Geometry: final body of the model. Coordinates: model frame, mm. A direction names the side the tool comes from. Give positions to 0.01 mm unless a question says otherwise; leave off trailing zeros. Loops run counter-clockwise (first coordinate to the right, second up) from the corner with the lowest first, then second, coordinate; pieces in that order, holes last. Notation, with made-up numbers: (27, 28.25) -> (85, 28.25) arc R3 cw to (85, 33.25) -> close; hole circle Ø7 at (1.5, 51.25). An arc over 180 degrees is marked (long way). One line per item, written item: value. Start each with the question number.
from build123d import *

# Parameters (mm, degrees)
F0_R     = 10.658227
F1_DEPTH = 76.2


with BuildPart() as f1:
    # F0 (on Front) → F1 (new body)
    with BuildSketch(Plane.XZ):
        Polygon((-47.944785, 43.843842), (-36.889297, 33.354142), (-22.277207, 37.683625), (-18.720605, 52.502808), (-29.776092, 62.992508), (-44.388182, 58.663024), align=None)
        with Locations((-33.332695, 48.173325)):
            Circle(F0_R, mode=Mode.SUBTRACT)
        Polygon((-40.4459, 18.534959), (-36.889297, 33.354142), (-47.944785, 43.843842), (-62.556875, 39.514358), (-66.113477, 24.695176), (-55.05799, 14.205476), align=None)
        with Locations((-51.501387, 29.024659)):
            Circle(F0_R, mode=Mode.SUBTRACT)
        Polygon((-22.277207, 37.683625), (-36.889297, 33.354142), (-40.4459, 18.534959), (-29.390412, 8.04526), (-14.778322, 12.374743), (-11.22172, 27.193926), align=None)
        with Locations((-25.83381, 22.864443)):
            Circle(F0_R, mode=Mode.SUBTRACT)
        Polygon((-29.390412, 8.04526), (-40.4459, 18.534959), (-55.05799, 14.205476), (-58.614592, -0.613707), (-47.559105, -11.103406), (-32.947015, -6.773923), align=None)
        with Locations((-44.002502, 3.715776)):
            Circle(F0_R, mode=Mode.SUBTRACT)
        Polygon((-14.778322, 12.374743), (-29.390412, 8.04526), (-32.947015, -6.773923), (-21.891527, -17.263623), (-7.279437, -12.934139), (-3.722835, 1.885043), align=None)
        with Locations((-18.334925, -2.44444)):
            Circle(F0_R, mode=Mode.SUBTRACT)
        Polygon((3.39037, 31.523409), (-11.22172, 27.193926), (-14.778322, 12.374743), (-3.722835, 1.885043), (10.889255, 6.214527), (14.445858, 21.03371), align=None)
        with Locations((-0.166232, 16.704226)):
            Circle(F0_R, mode=Mode.SUBTRACT)
        Polygon((-18.720605, 52.502808), (-22.277207, 37.683625), (-11.22172, 27.193926), (3.39037, 31.523409), (6.946973, 46.342592), (-4.108515, 56.832291), align=None)
        with Locations((-7.665117, 42.013109)):
            Circle(F0_R, mode=Mode.SUBTRACT)
    extrude(amount=F1_DEPTH)


solid = f1.part
Item 1: Section D-D, the plane x = 1.5. Output: boundary loops of the cut face in (y, z), then the cut area to 3 significant figures.
Item 2: Section C-C, the plane x = -16.5. Output: boundary loops of the cut face in (y, z), then the cut area to 3 significant figures.
Item 3: Section A-A, the plane z = 9.5. Output: boundary loops of the cut face in (x, y), then the cut area to 3 significant figures.
Item 4: Section B-B, the plane y = -51.5. Output: boundary loops of the cut face in (x, z), then the cut area to 3 significant figures.
Item 5: Access query for faces 1 (the face through (-40.36, -37.57, -8.97)), 2 (the face through (-46.14, -37.57, 51.36)), 3 (the face through (-11.3, -37.6, 54.7)), 4 (the face through (5.144, -37.567, 38.829)). Directions: +Z, -Z, +X, -X, +Y, -Y. A direction counts if a zero-diameter tool reaches every point of the face in a straight line with its end or side. Return the directions, or none.
Item 6: Pin query (flat end, axial travel): pin 1 (6 mm diameter, centred on x = -57.5, y = -52, fed in from -Z); pin 2 (3 mm diameter, centred on x = -33, y = -8.5, fed in from +Z); pin 3 (1.5 mm diameter, centred on y = -68, z = 13, fed in from -X). Return the tip coordinate at first contact, or that it passes through.
Item 7: Ray query, line 1 along X through (y, z) = (-26, 29.5); line 2 along X through (y, z) = (-21, -2); line 3 along Z through (x, y) = (-22.5, -62.5). Return the intervals inside material, ascending. Write a range as [from, to].
Item 8: Mould query, pull axis Z, two halves, no side actions, for faces 5 (the face through (9, -37.6, 26.2)), 6 (the face through (-35, -76.2, 29)), 7 (the face through (3.48, -37.57, 4.02)), 8 (the face through (-64.31, -37.57, 32.21)). Classes: pulls with the +Z half, pulls with the -Z half, needs draft (parallel to the pull), parting line crosses it, or undercut.
Geometry check:
1. outline: (-76.2, 3.43) -> (0, 3.43) -> (0, 6.18) -> (-76.2, 6.18) -> close; (-76.2, 27.23) -> (0, 27.23) -> (0, 36.57) -> (-76.2, 36.57) -> close; (-76.2, 47.45) -> (0, 47.45) -> (0, 51.51) -> (-76.2, 51.51) -> close
1. area: 1,230 mm2
2. outline: (-76.2, -15.67) -> (0, -15.67) -> (0, -12.94) -> (-76.2, -12.94) -> close; (-76.2, 8.05) -> (0, 8.05) -> (0, 17.72) -> (-76.2, 17.72) -> close; (-76.2, 28.01) -> (0, 28.01) -> (0, 36.05) -> (-76.2, 36.05) -> close; (-76.2, 47.97) -> (0, 47.97) -> (0, 53.16) -> (-76.2, 53.16) -> close
2. area: 1,950 mm2
3. outline: (-56.19, -76.2) -> (-52.95, -76.2) -> (-52.95, 0) -> (-56.19, 0) -> close; (-35.05, -76.2) -> (-8.02, -76.2) -> (-8.02, 0) -> (-35.05, 0) -> close; (7.69, -76.2) -> (11.68, -76.2) -> (11.68, 0) -> (7.69, 0) -> close
3. area: 2,610 mm2
4. outline: (-66.11, 24.7) -> (-55.06, 14.21) -> (-58.61, -0.61) -> (-47.56, -11.1) -> (-32.95, -6.77) -> (-21.89, -17.26) -> (-7.28, -12.93) -> (-3.72, 1.89) -> (10.89, 6.21) -> (14.45, 21.03) -> (3.39, 31.52) -> (6.95, 46.34) -> (-4.11, 56.83) -> (-18.72, 52.5) -> (-29.78, 62.99) -> (-44.39, 58.66) -> (-47.94, 43.84) -> (-62.56, 39.51) -> close; hole circle Ø21.32 at (-51.5, 29.02); hole circle Ø21.32 at (-44, 3.72); hole circle Ø21.32 at (-33.33, 48.17); hole circle Ø21.32 at (-25.83, 22.86); hole circle Ø21.32 at (-18.33, -2.44); hole circle Ø21.32 at (-7.67, 42.01); hole circle Ø21.32 at (-0.17, 16.7)
4. area: 1,730 mm2
5. face 1: -Z, +Y, -Y
5. face 2: +Z, -X, +Y, -Y
5. face 3: +Z, +Y, -Y
5. face 4: +X, +Y, -Y
6. pin 1: stops at z = -4.52
6. pin 2: stops at z = 62.48
6. pin 3: stops at x = -55.53
7. line 1: x = [-64.96, -62.15], [-40.85, -34.17], [-17.49, 5.52]
7. line 2: x = [-57.15, -53], [-35.01, -28.98], [-7.69, -4.66]
7. line 3: z = [-16.69, -12.26], [7.37, 12.74], [32.99, 56.09]
8. face 5: undercut
8. face 6: needs draft
8. face 7: pulls with the -Z half
8. face 8: pulls with the +Z half
